Work out the finished part from the listing and answer in its coordinate system (mm). A direction names the side the tool comes from. Round coordinates to 2 decimals unless told otherwise and drop trailing zeros. Order: outer loops, then holes, each group sorted by start corner. A loop starts at its lowest first (then second) coordinate and runs counter-clockwise, first axis right, second up. Notation, with made-up numbers: (-32, 81.25) - (19, 81.25) arc R13 ccw to (19, 85.25) - close; hole circle Ø6 at (59.25, 0.5). An arc over 180 degrees is marked (long way). Use one line per item in the form item = value. Start each with the question number.
Q1. For a pull along X with two mould halves and no side action, classify faces 3 (the flat face through (-151.027, -268.753, 4.93)), 4 (the flat face through (159.21, -262, 4.93)), 5 (the cylindrical face through (1.03, 59.99, 4.93)), 6 (the flat face through (-110, -152, 0)) as +X half, -X half, draft (parallel to the pull), parting line (faces both ways), or undercut.
Q2. The part is cut by section A-A on z = 2. Determine the outline of the cut face in (x, y), plus the area to 3 significant figures.
Q3. The part is cut by section C-C on x = -17. Determine the outline of the cut face in (y, z), plus the area to 3 significant figures.
Q4. Which of the six approach directions +Z, -Z, +X, -X, +Y, -Y give full straight-line access (tool end or side, diameter ignored) to faces 1 (the flat face through (-110, -152, 10)), 2 (the flat face through (148.154, -260.86, 4.93))?
Q5. The part is cut by section D-D on x = 230. Determine the outline of the cut face in (y, z), plus the area to 3 significant figures.
Q6. Given P1, Ø4, axis at y = -2, z = 1, coming from the -X side; P2, Ø3, axis at x = 274.5, z = 3.5, coming from the +Y side; P3, Ø1, axis at y = -14.5, z = 5, coming from the +X side, each flat-ended and moving along its own axis, determine where each tip first touches the part or whether it passes through.
Q7. The part is cut by section B-B on y = -482. Determine the outline of the cut face in (x, z).
Q8. Find the intervals of material crossed by line 1 (X direction, y = -37.5, z = 9.75); line 2 (Y direction, x = 269, z = 1); line 3 (X direction, y = -317, z = 6), in increasing order. Write a range as [from, to].
from build123d import *

# Parameters (mm, degrees)
EXTRUDE_1_DEPTH = 10


with BuildPart() as part:
    # Эскиз1 → Бобышка-Вытянуть1 (new body)
    with BuildSketch(Plane.XY):
        with BuildLine():
            Line((-292.196717035, -546.714565305), (-252.196717035, -546.714565305))
            Line((-252.196717035, -546.714565305), (-46.984631039, 17.101007166))
            ThreePointArc((-46.984631039, 17.101007166), (0, 50), (46.984631039, 17.101007166))
            Line((46.984631039, 17.101007166), (252.196717035, -546.714565305))
            Line((252.196717035, -546.714565305), (292.196717035, -546.714565305))
            Line((292.196717035, -546.714565305), (292.196717035, -536.714565305))
            Line((292.196717035, -536.714565305), (259.198792417, -536.714565305))
            Line((259.198792417, -536.714565305), (56.381557247, 20.5212086))
            ThreePointArc((56.381557247, 20.5212086), (0, 60), (-56.381557247, 20.5212086))
            Line((-56.381557247, 20.5212086), (-259.198792417, -536.714565305))
            Line((-259.198792417, -536.714565305), (-292.196717035, -536.714565305))
            Line((-292.196717035, -536.714565305), (-292.196717035, -546.714565305))
        make_face()
    extrude(amount=EXTRUDE_1_DEPTH)


solid = part.part
Found:
q1.face_3 = undercut
q1.face_4 = +X half
q1.face_5 = parting line
q1.face_6 = draft
q2.outline = (-292.2, -546.71) - (-252.2, -546.71) - (-46.98, 17.1) arc R50 cw to (46.98, 17.1) - (252.2, -546.71) - (292.2, -546.71) - (292.2, -536.71) - (259.2, -536.71) - (56.38, 20.52) arc R60 ccw to (-56.38, 20.52) - (-259.2, -536.71) - (-292.2, -536.71) - close
q2.area = 14,000 mm²
q3.outline = (47.02, 0) - (57.54, 0) - (57.54, 10) - (47.02, 10) - close
q3.area = 105 mm²
q4.face_1 = +Z, +X, -X, +Y, -Y
q4.face_2 = +Z, -Z, -Y
q5.outline = (-485.73, 0) - (-456.49, 0) - (-456.49, 10) - (-485.73, 10) - close
q5.area = 292 mm²
q6.P1 = -65.31
q6.P2 = -536.71
q6.P3 = 69.31
q7.outline = (-239.28, 0) - (-228.64, 0) - (-228.64, 10) - (-239.28, 10) - close; (228.64, 0) - (239.28, 0) - (239.28, 10) - (228.64, 10) - close
q8.line_1 = [-77.5, -66.86], [66.86, 77.5]
q8.line_2 = [-546.71, -536.71]
q8.line_3 = [-179.23, -168.59], [168.59, 179.23]
